Check sheet for the modelled part. Datum: model origin and axes. Units: mm. Face numbers are marked on the shaded views. Round coordinates to 2 decimals unless told otherwise and drop trailing zeros. Write each loop counter-clockwise with the first axis right and the second up, starting at its lowest first coordinate (ties: lowest second). Pieces come first, ordered by that corner, then holes. Notation, with made-up numbers: (-36.75, 28.25) -> (15.25, 28.25) arc R25 ccw to (15.25, 55.25) -> close; hole circle Ø3 at (22.5, 64). An arc over 180 degrees is marked (long way). Write item = value, one per line.
from build123d import *

# Parameters (mm, degrees)
F2_DEPTH = 7
F0_R     = 11.5
F3_DEPTH = 26.416


with BuildPart() as f2:
    # F1 (on Front) → F2 (new body)
    with BuildSketch(Plane.XZ):
        with BuildLine():
            ThreePointArc((-9.8594943471, 13.4371291696), (-9.8598798703, 13.3389562022), (-9.8610364161, 13.2407892906))
            Line((-9.8610364161, 13.2407892906), (-9.5237098666, 13.2354901845))
            Line((-9.5237098666, 13.2354901845), (-9.4420993874, 13.234208155))
            Line((-9.4420993874, 13.234208155), (-8.9874716534, 14.0291067183))
            ThreePointArc((-8.9874716534, 14.0291067183), (-33.8655402549, 20.2761595034), (-16.4893494105, 1.4078803666))
            Line((-16.4893494105, 1.4078803666), (-15.9845189072, 2.2945213217))
            Line((-15.9845189072, 2.2945213217), (-16.1520543214, 2.5873509079))
            ThreePointArc((-16.1520543214, 2.5873509079), (-33.1725189083, 19.7083730525), (-9.8594943471, 13.4371291696))
        make_face()
        with BuildLine():
            Line((-15.7125081445, 1.8190827434), (-15.9845189072, 2.2945213217))
            Line((-15.9845189072, 2.2945213217), (-16.4893494105, 1.4078803666))
            ThreePointArc((-16.4893494105, 1.4078803666), (-16.0975525686, 1.6071032397), (-15.7125081445, 1.8190827434))
        make_face()
        with BuildLine():
            Line((-8.9874716534, 14.0291067183), (-9.4420993874, 13.234208155))
            Line((-9.4420993874, 13.234208155), (-8.9760259484, 13.2268865476))
            ThreePointArc((-8.9760259484, 13.2268865476), (-8.974787508, 13.3320046163), (-8.9743746861, 13.4371291696))
            ThreePointArc((-8.9743746861, 13.4371291696), (-8.9776493285, 13.7331903747), (-8.9874716534, 14.0291067183))
        make_face()
        with BuildLine():
            Line((-6.6469862026, -14.026241978), (-15.7125081445, 1.8190827434))
            ThreePointArc((-15.7125081445, 1.8190827434), (-16.0975525686, 1.6071032397), (-16.4893494105, 1.4078803666))
            Line((-16.4893494105, 1.4078803666), (-25.3977489889, -14.2380678461))
            Line((-25.3977489889, -14.2380678461), (-7.3951647118, -14.4875430354))
            ThreePointArc((-7.3951647118, -14.4875430354), (-7.0248630052, -14.2507495292), (-6.6469862026, -14.026241978))
        make_face()
        with BuildLine():
            ThreePointArc((-8.9743746861, 13.4371291696), (-8.974787508, 13.3320046163), (-8.9760259484, 13.2268865476))
            Line((-8.9760259484, 13.2268865476), (8.9760259484, 12.9448754613))
            ThreePointArc((8.9760259484, 12.9448754613), (8.989763273, 13.3762864413), (9.0174033464, 13.8070301865))
            Line((9.0174033464, 13.8070301865), (-0.1233932709, 29.5275962356))
            Line((-0.1233932709, 29.5275962356), (-8.9874716534, 14.0291067183))
            ThreePointArc((-8.9874716534, 14.0291067183), (-8.9776493285, 13.7331903747), (-8.9743746861, 13.4371291696))
        make_face()
        with BuildLine():
            Line((-6.3749754398, -14.5016805563), (-6.6469862026, -14.026241978))
            ThreePointArc((-6.6469862026, -14.026241978), (-7.0248630052, -14.2507495292), (-7.3951647118, -14.4875430354))
            Line((-7.3951647118, -14.4875430354), (-6.3749754398, -14.5016805563))
        make_face()
        with BuildLine():
            ThreePointArc((9.0174033464, 13.8070301865), (8.989763273, 13.3762864413), (8.9760259484, 12.9448754613))
            Line((8.9760259484, 12.9448754613), (9.5237098666, 12.9362718244))
            Line((9.5237098666, 12.9362718244), (9.0174033464, 13.8070301865))
        make_face()
        with BuildLine():
            Line((-6.2074400257, -14.7945101426), (-6.3749754398, -14.5016805563))
            Line((-6.3749754398, -14.5016805563), (-7.3951647118, -14.4875430354))
            ThreePointArc((-7.3951647118, -14.4875430354), (-6.3315189236, -37.4372225794), (13.385119661, -25.6442884042))
            ThreePointArc((13.385119661, -25.6442884042), (11.825746284, -19.3742682156), (7.5109617661, -14.5651692295))
            Line((7.5109617661, -14.5651692295), (6.4622937408, -14.5520938009))
            Line((6.4622937408, -14.5520938009), (6.2924635872, -14.8435985187))
            ThreePointArc((6.2924635872, -14.8435985187), (10.8375687965, -19.415556384), (12.5, -25.6442884042))
            ThreePointArc((12.5, -25.6442884042), (-6.2712438829, -36.4573129654), (-6.2074400257, -14.7945101426))
        make_face()
        with BuildLine():
            ThreePointArc((7.5109617661, -14.5651692295), (7.1286450726, -14.3153940288), (6.7380302462, -14.0788062811))
            Line((6.7380302462, -14.0788062811), (6.4622937408, -14.5520938009))
            Line((6.4622937408, -14.5520938009), (7.5109617661, -14.5651692295))
        make_face()
        with BuildLine():
            Line((15.6214641009, 1.1691507162), (6.7380302462, -14.0788062811))
            ThreePointArc((6.7380302462, -14.0788062811), (7.1286450726, -14.3153940288), (7.5109617661, -14.5651692295))
            Line((7.5109617661, -14.5651692295), (25.4854150726, -14.7892856087))
            Line((25.4854150726, -14.7892856087), (16.4257602341, 0.7366235122))
            ThreePointArc((16.4257602341, 0.7366235122), (16.0199223632, 0.9460258224), (15.6214641009, 1.1691507162))
        make_face()
        with BuildLine():
            Line((9.0174033464, 13.8070301865), (9.5237098666, 12.9362718244))
            Line((9.5237098666, 12.9362718244), (9.8610364161, 12.9309727184))
            ThreePointArc((9.8610364161, 12.9309727184), (22.4576673144, 25.2342473162), (34.8594943471, 12.7346328394))
            ThreePointArc((34.8594943471, 12.7346328394), (28.5882263673, 1.8970640428), (16.0670307599, 1.9339429538))
            Line((16.0670307599, 1.9339429538), (15.8972006063, 1.642438236))
            Line((15.8972006063, 1.642438236), (16.4257602341, 0.7366235122))
            ThreePointArc((16.4257602341, 0.7366235122), (29.4212819112, 1.363943118), (35.7446140081, 12.7346328394))
            ThreePointArc((35.7446140081, 12.7346328394), (22.8961244654, 26.1089910092), (9.0174033464, 13.8070301865))
        make_face()
        with BuildLine():
            Line((15.8972006063, 1.642438236), (15.6214641009, 1.1691507162))
            ThreePointArc((15.6214641009, 1.1691507162), (16.0199223632, 0.9460258224), (16.4257602341, 0.7366235122))
            Line((16.4257602341, 0.7366235122), (15.8972006063, 1.642438236))
        make_face()
        with BuildLine():
            Line((-9.5237098666, 13.2354901845), (-9.8610364161, 13.2407892906))
            ThreePointArc((-9.8610364161, 13.2407892906), (-11.5960566093, 7.0811549669), (-16.1520543214, 2.5873509079))
            Line((-16.1520543214, 2.5873509079), (-15.9845189072, 2.2945213217))
            Line((-15.9845189072, 2.2945213217), (-15.7125081445, 1.8190827434))
            ThreePointArc((-15.7125081445, 1.8190827434), (-10.8339021804, 6.6310911483), (-8.9760259484, 13.2268865476))
            Line((-8.9760259484, 13.2268865476), (-9.4420993874, 13.234208155))
            Line((-9.4420993874, 13.234208155), (-9.5269323957, 13.0858810045))
            ThreePointArc((-9.5269323957, 13.0858810045), (-9.5251031319, 13.1606808989), (-9.5237098666, 13.2354901845))
        make_face()
        with BuildLine():
            ThreePointArc((6.7380302462, -14.0788062811), (0.0525643031, -12.2592719555), (-6.6469862026, -14.026241978))
            Line((-6.6469862026, -14.026241978), (-6.3749754398, -14.5016805563))
            Line((-6.3749754398, -14.5016805563), (-6.2074400257, -14.7945101426))
            ThreePointArc((-6.2074400257, -14.7945101426), (0.0490883761, -13.1443847914), (6.2924635872, -14.8435985187))
            Line((6.2924635872, -14.8435985187), (6.4622937408, -14.5520938009))
            Line((6.4622937408, -14.5520938009), (6.7380302462, -14.0788062811))
        make_face()
        with BuildLine():
            ThreePointArc((-8.9760259484, 13.2268865476), (-10.8339021804, 6.6310911483), (-15.7125081445, 1.8190827434))
            Line((-15.7125081445, 1.8190827434), (-6.6469862026, -14.026241978))
            ThreePointArc((-6.6469862026, -14.026241978), (0.0525643031, -12.2592719555), (6.7380302462, -14.0788062811))
            Line((6.7380302462, -14.0788062811), (15.6214641009, 1.1691507162))
            ThreePointArc((15.6214641009, 1.1691507162), (10.7024964382, 6.15619624), (8.9760259484, 12.9448754613))
            Line((8.9760259484, 12.9448754613), (-8.9760259484, 13.2268865476))
        make_face()
        with BuildLine():
            Line((9.5237098666, 12.9362718244), (8.9760259484, 12.9448754613))
            ThreePointArc((8.9760259484, 12.9448754613), (10.7024964382, 6.15619624), (15.6214641009, 1.1691507162))
            Line((15.6214641009, 1.1691507162), (15.8972006063, 1.642438236))
            Line((15.8972006063, 1.642438236), (16.0670307599, 1.9339429538))
            ThreePointArc((16.0670307599, 1.9339429538), (11.4733403529, 6.5912094278), (9.8610364161, 12.9309727184))
            Line((9.8610364161, 12.9309727184), (9.5237098666, 12.9362718244))
        make_face()
    extrude(amount=F2_DEPTH)

    # F0 (on Front) → F3 (cut)
    with BuildSketch(Plane.XZ):
        Circle(F0_R)
    extrude(amount=F3_DEPTH, mode=Mode.SUBTRACT)


solid = f2.part
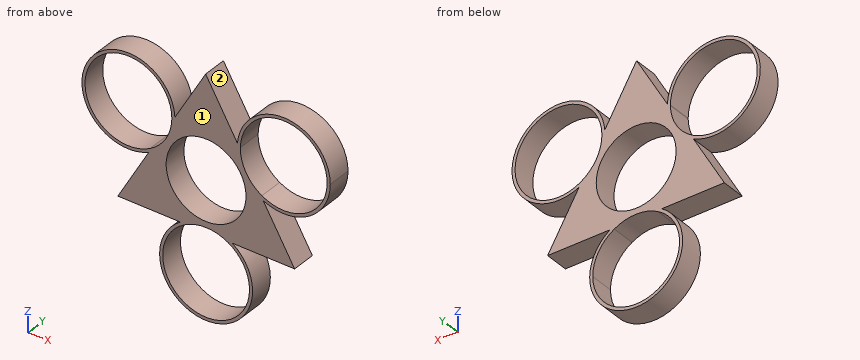
(1) Material ranges on L1, parallel to Z at x = -17.5, y = -4.5; L2, parallel to Z at x = -24, y = -6; L3, parallel to X at y = -2, z = 22, recorded low to high. Write a range as [from, to].
Worked answers:
L1 = [-14.35, -0.37], [0.97, 1.92], [24.95, 25.91]
L2 = [-14.26, -11.78], [0.15, 1.05], [25.83, 26.72]
L3 = [-32.65, -31.47], [-13.25, -12.07], [-4.43, 4.25], [12.7, 13.97], [30.75, 32.02]
(2) Release check for a two-part mould opening along X. For the marked faces 1 and 2 record: pulls with the +X half, pulls with the -X half, needs draft (parallel to the pull), parting line crosses it, or undercut.
Worked answers:
face_1 = needs draft
face_2 = undercut
(3) Sectioned sample at C-C on z = 21.5. Enter the section's corners in (x, y).
Worked answers:
outline = (-33.04, -7) -> (-31.91, -7) -> (-31.91, 0) -> (-33.04, 0) -> close; (-12.81, -7) -> (-11.68, -7) -> (-11.68, 0) -> (-12.81, 0) -> close; (-4.71, -7) -> (4.54, -7) -> (4.54, 0) -> (-4.71, 0) -> close; (12.24, -7) -> (13.45, -7) -> (13.45, 0) -> (12.24, 0) -> close; (31.27, -7) -> (32.48, -7) -> (32.48, 0) -> (31.27, 0) -> close
(4) Sectioned sample at B-B on z = -19. Enter the section's corners in (x, y), then the cut area to 3 significant figures.
Worked answers:
outline = (-11.62, -7) -> (-10.59, -7) -> (-10.59, 0) -> (-11.62, 0) -> close; (10.59, -7) -> (11.62, -7) -> (11.62, 0) -> (10.59, 0) -> close
area = 14.4 mm²
(5) Sectioned sample at A-A on y = -2.25. Enter the section's corners in (x, z).
Worked answers:
outline = (-25.4, -14.24) -> (-7.4, -14.49) arc R13.39 ccw (long way) to (7.51, -14.57) -> (25.49, -14.79) -> (16.43, 0.74) arc R13.39 ccw (long way) to (9.02, 13.81) -> (-0.12, 29.53) -> (-8.99, 14.03) arc R13.39 ccw (long way) to (-16.49, 1.41) -> close; hole circle Ø25 at (-22.36, 13.44); hole circle Ø25 at (0, -25.64); hole circle Ø23 at (0, 0); hole (-9.53, 13.09) -> (-9.44, 13.23) -> (-9.52, 13.24) arc R12.84 cw to start; hole circle Ø25 at (22.36, 12.73)
(6) Go/stop test with flat-tipped pins: P1, Ø20.5, axis at x = 0, z = 0, coming from the +Y side; P2, Ø1.5, axis at y = -2.5, z = -7.5, coming from the +X side; P3, Ø3, axis at y = -5.5, z = -24.5, coming from the +X side; P4, Ø4, axis at x = 12, y = -1.5, coming from the -Z side. Record where each tip stops, or that it passes through.
Worked answers:
P1 = through
P2 = 21.67
P3 = 13.39
P4 = -34.54
